Autodesk Inventor part; units mm, degrees
ref_plane "YZ Plane" through (0, 0, 0) normal (1, 0, 0) x (0, 1, 0)
ref_plane "XZ Plane" through (0, 0, 0) normal (0, 1, 0) x (-1, 0, 0)
ref_plane "XY Plane" through (0, 0, 0) normal (0, 0, 1) x (1, 0, 0)
sketch "Sketch1" plane through (0, 0, 0) normal (0, 0, 1) x (1, 0, 0)
  line L0 (0, 0) -> (10.4, 0)
  line L1 (10.4, 0) -> (10.4, 13.4)
  line L2 (10.4, 13.4) -> (0, 13.4)
  line L3 (0, 13.4) -> (0, 0)
  dimension "d0" = 10.4
  dimension "d1" = 13.4
extrude "Extrusion1" add sketch "Sketch1" along normal blind 1.6
sketch "Sketch2" plane through (0, 0, 1.6) normal (0, 0, 1) x (1, 0, 0)
  line L0 (10.4, 13.4) -> (0, 13.4)
  line L1 (0, 13.4) -> (0, 0)
  point P0 (2.7, 10.6)
  dimension "d4" = 2.8
  dimension "d5" = 2.7
hole "Hole1" at (2.7, 10.6, 1.6) direction (0, 0, -1) diameter 3 depth 1.6
sketch "Sketch3" plane through (0, 0, 1.6) normal (0, 0, 1) x (1, 0, 0)
  line L0 (0, 13.4) -> (0, 0)
  line L1 (10.4, 0) -> (10.4, 13.4)
  line L2 (0, 0) -> (10.4, 0)
  point P0 (1.39, 1)
  point P1 (3.93, 1)
  point P2 (6.47, 1)
  point P3 (9.01, 1)
  point P4 (6.56, 11.8363)
  point P5 (9.1, 11.8363)
  dimension "d13" = 2.54
  dimension "d14" = 2.54
  dimension "d15" = 2.54
  dimension "d16" = 1.39
  dimension "d17" = 2.54
  dimension "d18" = 1.3
  dimension "d19" = 1
hole "Hole2" at (1.39, 1, 1.6) at (3.93, 1, 1.6) at (6.47, 1, 1.6) at (9.01, 1, 1.6) at (6.56, 11.8363, 1.6) at (9.1, 11.8363, 1.6) direction (0, 0, -1) diameter 1 end through all
sketch "Sketch4" plane through (0, 0, 1.6) normal (0, 0, 1) x (1, 0, 0)
  line L0 (5.4, 7.9) -> (9.9, 7.9)
  line L1 (9.9, 7.9) -> (9.9, 10.2)
  line L2 (9.9, 10.2) -> (5.4, 10.2)
  line L3 (5.4, 10.2) -> (5.4, 7.9)
  line L4 (10.4, 0) -> (10.4, 13.4)
  line L5 (10.4, 13.4) -> (0, 13.4)
  point P0 (0, 0)
  dimension "d27" = 4.5
  dimension "d28" = 2.3
  dimension "d29" = 0.5
  dimension "d30" = 3.2
extrude "Extrusion2" add sketch "Sketch4" along normal blind 1
properties part number "vl53l0x"
Geometry check sheet. Reference: the model listing, model coordinates, mm. A direction names the side the tool comes from. Give positions to 0.01 mm unless a question says otherwise; leave off trailing zeros. Write each loop counter-clockwise with the first axis right and the second up, starting at its lowest first coordinate (ties: lowest second). Pieces come first, ordered by that corner, then holes.
1) Material ranges on L1, parallel to Y at x = 6.5, z = 1.2; L2, parallel to Y at x = 6.25, z = 0.6; L3, parallel to X at y = 10.6, z = 1.15, recorded low to high.
2) Section check D-D, the plane z = 2.35. Record the boundary of the cut face in (x, y), and give its area (4 significant figures).
3) Section check B-B, the plane x = 2.7. Record the boundary of the cut face in (y, z).
4) Release check for a two-part mould opening along X. For faces 4 (the flat face through (5.4, 9, 2)), 5 (the flat face through (10.4, 7, 1)), 6 (the cylindrical face through (9.292, 11.374, 0.789)), 7 (the flat face through (5, 13.4, 1)) record: pulls with the +X half, pulls with the -X half, needs draft (parallel to the pull), parting line crosses it, or undercut.
5) Section check A-A, the plane z = 0.85. Record the boundary of the cut face in (x, y), and give its area (3 significant figures).
6) Section check C-C, the plane x = 3.93. Record the boundary of the cut face in (y, z).
7) Gauge pin test, flat ends, axial feed: pin 1 (1.1 mm diameter, centred on x = 7, z = 2.5, fed in from -Y); pin 2 (5 mm diameter, centred on x = 5, y = 5, fed in from +Z). Record the tip position at first contact, or that the pin passes through.
8) Access from +Z, -Z, +X, -X, +Y, -Y to the whole of each face (thin tool, end or side, straight path). Record for faces 1 (the flat face through (8, 10.2, 2)), 2 (the flat face through (8, 7.9, 2)), 3 (the flat face through (9.9, 9, 2)).
Computed:
1. L1: y = 0 to 0.5, 1.5 to 11.34, 12.33 to 13.4
1. L2: y = 0 to 0.55, 1.45 to 11.44, 12.23 to 13.4
1. L3: x = 0 to 1.2, 4.2 to 10.4
2. outline: (5.4, 7.9) - (9.9, 7.9) - (9.9, 10.2) - (5.4, 10.2) - close
2. area: 10.35 mm2
3. outline: (0, 0) - (9.1, 0) - (9.1, 1.6) - (0, 1.6) - close; (12.1, 0) - (13.4, 0) - (13.4, 1.6) - (12.1, 1.6) - close
4. face 4: pulls with the -X half
4. face 5: pulls with the +X half
4. face 6: undercut
4. face 7: needs draft
5. outline: (0, 0) - (10.4, 0) - (10.4, 13.4) - (0, 13.4) - close; hole circle Ø1 at (1.39, 1); hole circle Ø3 at (2.7, 10.6); hole circle Ø1 at (3.93, 1); hole circle Ø1 at (6.47, 1); hole circle Ø1 at (6.56, 11.84); hole circle Ø1 at (9.01, 1); hole circle Ø1 at (9.1, 11.84)
5. area: 128 mm2
6. outline: (0, 0) - (0.5, 0) - (0.5, 1.6) - (0, 1.6) - close; (1.5, 0) - (9.74, 0) - (9.74, 1.6) - (1.5, 1.6) - close; (11.46, 0) - (13.4, 0) - (13.4, 1.6) - (11.46, 1.6) - close
7. pin 1: stops at y = 7.9
7. pin 2: stops at z = 1.6
8. face 1: +Z, +X, -X, +Y
8. face 2: +Z, +X, -X, -Y
8. face 3: +Z, +X, +Y, -Y
